Here's how the part is built. I have some questions about the finished solid (model axes, mm). A direction names the side the tool comes from. Round coordinates to 2 decimals unless told otherwise and drop trailing zeros. Order: outer loops, then holes, each group sorted by start corner. A loop starts at its lowest first (then second) coordinate and runs counter-clockwise, first axis right, second up. Notation, with made-up numbers: (-1.5, -21.5) -> (30.5, -21.5) arc R21 ccw to (30.5, 16.5) -> close; hole circle Ø9 at (73, 29). An arc over 180 degrees is marked (long way). Answer in a Markdown table with one row per item.
```python
from build123d import *

# Parameters (mm, degrees)
F0_R          = 18.013064
F1_DEPTH      = 50.8
F1_DEPTH_BACK = 50.8
F3_DEPTH      = 20.32
F5_DEPTH      = 20.32
F6_R          = 8.017692
F7_DEPTH      = 101.601


with BuildPart() as f1:
    # F0 (on Front) → F1 (new body, two sides)
    with BuildSketch(Plane.XZ) as f1_sk:
        Circle(F0_R)
    extrude(amount=F1_DEPTH)
    extrude(f1_sk.sketch, amount=-F1_DEPTH_BACK)

    # F2 (on face) → F3 (join)
    with BuildSketch(Plane.XZ.offset(50.8)):
        Polygon((-18.013064, 49.393319), (-18.013064, 0), (18.013064, 0), (18.013064, 49.393319), (0, 49.393319), align=None)
        with BuildLine():
            Line((18.013064, 0), (-18.013064, 0))
            ThreePointArc((-18.013064, 0), (0, -18.013064), (18.013064, 0))
        make_face()
        with BuildLine():
            ThreePointArc((18.013064, 49.393319), (0, 67.406383), (-18.013064, 49.393319))
            Line((-18.013064, 49.393319), (0, 49.393319))
            Line((0, 49.393319), (18.013064, 49.393319))
        make_face()
    extrude(amount=-F3_DEPTH)

    # F4 (on face) → F5 (join)
    with BuildSketch(Plane(origin=(0, 50.8, 0), x_dir=(-1, 0, 0), z_dir=(0, 1, 0))):
        Polygon((-17.788198, 49.871705), (-18.013064, 0), (18.013064, 0), (18.013064, 49.871705), align=None)
        with BuildLine():
            ThreePointArc((18.013064, 49.871705), (0.112433, 67.691806), (-17.788198, 49.871705))
            Line((-17.788198, 49.871705), (18.013064, 49.871705))
        make_face()
    extrude(amount=-F5_DEPTH)

    # F6 (on face) → F7 (cut, through all)
    with BuildSketch(Plane.XZ.offset(50.8)):
        Circle(F6_R)
        with Locations((-0.617001, 48.436549)):
            Circle(F6_R)
    extrude(amount=-F7_DEPTH, mode=Mode.SUBTRACT)


solid = f1.part
```
1. Suppose I cut it at D-D on z = 22. Write out the boundary of the cut face in (x, y), then the cut area to 3 significant figures.
Numbers:
| item | result |
|---|---|
| outline | (-18.01, -50.8) -> (18.01, -50.8) -> (18.01, -30.48) -> (-18.01, -30.48) -> close; (-18.01, 30.48) -> (17.91, 30.48) -> (17.91, 50.8) -> (-18.01, 50.8) -> close |
| area | 1,460 mm2 |
2. Please list where these lines run through material, in increasing order: line 1 along Y through (x, z) = (10, 35); line 2 along Z through (x, y) = (0, -29); line 3 along X through (y, z) = (40.5, 41).
Numbers:
| item | result |
|---|---|
| line 1 | y = -50.8 to -30.48, 30.48 to 50.8 |
| line 2 | z = -18.01 to -8.02, 8.02 to 18.01 |
| line 3 | x = -18.01 to -3.61, 2.38 to 17.83 |
3. Suppose I cut it at A-A on z = 31. Write out the boundary of the cut face in (x, y), then the cut area to 3 significant figures.
Numbers:
| item | result |
|---|---|
| outline | (-18.01, -50.8) -> (18.01, -50.8) -> (18.01, -30.48) -> (-18.01, -30.48) -> close; (-18.01, 30.48) -> (17.87, 30.48) -> (17.87, 50.8) -> (-18.01, 50.8) -> close |
| area | 1,460 mm2 |
4. For pin 1 Ø5 at (x, y) = (8.5, -21.5) entering from +Z; pin 2 Ø12 at (y, z) = (-20, 21.5) entering from -X; pin 3 Ø4 at (x, y) = (-10.5, -35.5) entering from -Z; pin 4 Ø14.5 at (x, z) = (-0.62, 48.44) entering from +Y, each with a flat end and sliding along its axis, tell me the tip position at first contact or that it passes through.
Numbers:
| item | result |
|---|---|
| pin 1 | stops at z = 16.98 |
| pin 2 | stops at x = -9.18 |
| pin 3 | stops at z = -15.88 |
| pin 4 | passes through |
5. Suppose I cut it at B-B on x = 0. Write out the boundary of the cut face in (y, z).
Numbers:
| item | result |
|---|---|
| outline | (-50.8, -18.01) -> (50.8, -18.01) -> (50.8, -8.02) -> (-50.8, -8.02) -> close; (-50.8, 8.02) -> (50.8, 8.02) -> (50.8, 40.44) -> (30.48, 40.44) -> (30.48, 18.01) -> (-30.48, 18.01) -> (-30.48, 40.44) -> (-50.8, 40.44) -> close; (-50.8, 56.43) -> (-30.48, 56.43) -> (-30.48, 67.41) -> (-50.8, 67.41) -> close; (30.48, 56.43) -> (50.8, 56.43) -> (50.8, 67.69) -> (30.48, 67.69) -> close |
6. For faces 5 (the face through (18.013, -41, 24)), 6 (the face through (8.31, -0.71, -15.98)), which set-ups out of +Z, -Z, +X, -X, +Y, -Y let a thin tool reach every point of the face, with its end or its side?
Numbers:
| item | result |
|---|---|
| face 5 | +Z, -Z, +X, +Y, -Y |
| face 6 | none |
7. Suppose I cut it at C-C on y = -7. Write out the boundary of the cut face in (x, z).
Numbers:
| item | result |
|---|---|
| outline | circle Ø36.03 at (0, 0); hole circle Ø16.04 at (0, 0) |
8. We'd pull the mould along Z, two halves only. Please class faces 1 (the face through (-18.013, -41, 25)), 2 (the face through (7.647, -0.711, 2.408)), 3 (the face through (0.4, -40.8, 67.4)), 4 (the face through (-2.36, 40.5, 40.61)): released by +Z, released by -Z, zero draft, split by the parting line, or undercut.
Numbers:
| item | result |
|---|---|
| face 1 | zero draft |
| face 2 | undercut |
| face 3 | released by +Z |
| face 4 | undercut |
